Geometry: final body of the model. Coordinates: model frame, mm. Face numbers are marked on the shaded views. Coordinates: 2 decimals unless noted, no trailing zeros. Order: outer loops, then holes, each group sorted by start corner. A loop starts at its lowest first (then second) coordinate and runs counter-clockwise, first axis right, second up. Notation, with made-up numbers: M 25.25,0 L 34.25,0 A12 cw 34.25,18 Z; hole C 76.25,3 d3. An arc over 180 degrees is marked long. Write item = value, one per line.
from build123d import *

# Parameters (mm, degrees)
BOSS_EXTRUDE3_DEPTH = 7.8
SKETCH2_R           = 2.4
CUT_EXTRUDE1_DEPTH  = 7.8
SKETCH3_R           = 3.05
CUT_EXTRUDE2_DEPTH  = 0.8
SKETCH4_R           = 3.05
CUT_EXTRUDE3_DEPTH  = 0.8


with BuildPart() as part:
    # Sketch1 → Boss-Extrude3 (new body)
    with BuildSketch(Plane(origin=(0, 0, 0), x_dir=(1, 0, 0), z_dir=(0, 1, 0))):
        with BuildLine():
            Line((-16, -3.7), (32, -3.7))
            ThreePointArc((32, -3.7), (35.7, 0), (32, 3.7))
            Line((32, 3.7), (-16, 3.7))
            ThreePointArc((-16, 3.7), (-19.7, 0), (-16, -3.7))
        make_face()
    extrude(amount=BOSS_EXTRUDE3_DEPTH)

    # Sketch2 → Cut-Extrude1 (cut)
    with BuildSketch(Plane(origin=(0, 7.8, 0), x_dir=(1, 0, 0), z_dir=(0, 1, 0))):
        Circle(SKETCH2_R)
        with Locations((8, 0)):
            Circle(SKETCH2_R)
        with Locations((16, 0)):
            Circle(SKETCH2_R)
        with Locations((-16, 0)):
            Circle(SKETCH2_R)
        with Locations((-8, 0)):
            Circle(SKETCH2_R)
        with Locations((24, 0)):
            Circle(SKETCH2_R)
        with Locations((32, 0)):
            Circle(SKETCH2_R)
    extrude(amount=-CUT_EXTRUDE1_DEPTH, mode=Mode.SUBTRACT)

    # Sketch3 → Cut-Extrude2 (cut)
    with BuildSketch(Plane(origin=(0, 7.8, 0), x_dir=(1, 0, 0), z_dir=(0, 1, 0))):
        Circle(SKETCH3_R)
        with Locations((8, 0)):
            Circle(SKETCH3_R)
        with Locations((16, 0)):
            Circle(SKETCH3_R)
        with Locations((-16, 0)):
            Circle(SKETCH3_R)
        with Locations((-8, 0)):
            Circle(SKETCH3_R)
        with Locations((32, 0)):
            Circle(SKETCH3_R)
        with Locations((24, 0)):
            Circle(SKETCH3_R)
    extrude(amount=-CUT_EXTRUDE2_DEPTH, mode=Mode.SUBTRACT)

    # Sketch4 → Cut-Extrude3 (cut)
    with BuildSketch(Plane.XZ):
        Circle(SKETCH4_R)
        with Locations((8, 0)):
            Circle(SKETCH4_R)
        with Locations((16, 0)):
            Circle(SKETCH4_R)
        with Locations((-16, 0)):
            Circle(SKETCH4_R)
        with Locations((-8, 0)):
            Circle(SKETCH4_R)
        with Locations((32, 0)):
            Circle(SKETCH4_R)
        with Locations((24, 0)):
            Circle(SKETCH4_R)
    extrude(amount=-CUT_EXTRUDE3_DEPTH, mode=Mode.SUBTRACT)


solid = part.part
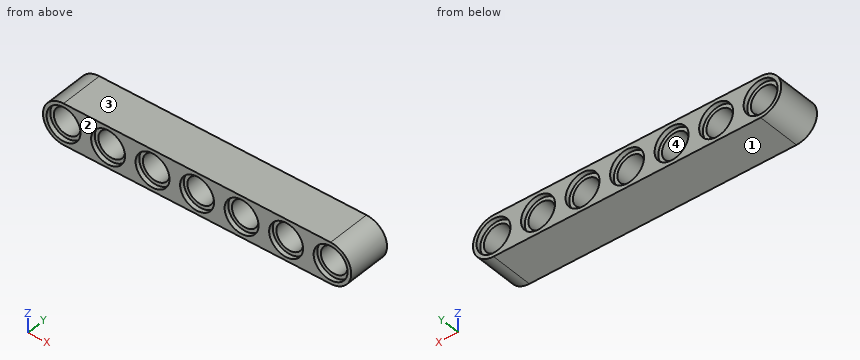
1) Mould query, pull axis Z, two halves, no side actions, for the marked faces 1, 2, 3 and 4. Classes: pulls with the +Z half, pulls with the -Z half, needs draft (parallel to the pull), parting line crosses it, or undercut.
Numbers:
face_1 = pulls with the -Z half
face_2 = needs draft
face_3 = pulls with the +Z half
face_4 = undercut
2) Section A-A, the plane y = 5.75. Return loops of the section in (x, z).
Numbers:
outline = M -16,-3.7 L 32,-3.7 A3.7 ccw 32,3.7 L -16,3.7 A3.7 ccw Z; hole C -16,0 d4.8; hole C -8,0 d4.8; hole C 0,0 d4.8; hole C 8,0 d4.8; hole C 16,0 d4.8; hole C 24,0 d4.8; hole C 32,0 d4.8
3) Section D-D, the plane x = 1. Return loops of the section in (y, z).
Numbers:
outline = M 0,-3.7 L 7.8,-3.7 L 7.8,-2.88 L 7,-2.88 L 7,-2.18 L 0.8,-2.18 L 0.8,-2.88 L 0,-2.88 Z; M 0,2.88 L 0.8,2.88 L 0.8,2.18 L 7,2.18 L 7,2.88 L 7.8,2.88 L 7.8,3.7 L 0,3.7 Z
4) Line query: L1, parallel to Z at x = 0, y = 7.45; L2, parallel to Z at x = 8, y = 1.5; L3, parallel to Y at x = -15, z = -2.5. Output: solid intervals per line, ascending.
Numbers:
L1 = -3.7 to -3.05, 3.05 to 3.7
L2 = -3.7 to -2.4, 2.4 to 3.7
L3 = 0.8 to 7
5) Pin query (flat end, axial travel): pin 1 (1 mm diameter, centred on y = 1.5, z = -1, fed in from +X); pin 2 (1.5 mm diameter, centred on y = 7, z = 1.5, fed in from +X); pin 3 (3 mm diameter, centred on y = 5, z = 2.5, fed in from -X). Return the tip coordinate at first contact, or that it passes through.
Numbers:
pin_1 = 35.67
pin_2 = 35.62
pin_3 = -19.56
6) Section B-B, the plane x = 24. Return loops of the section in (y, z), and give its area (3 significant figures).
Numbers:
outline = M 0,-3.7 L 7.8,-3.7 L 7.8,-3.05 L 7,-3.05 L 7,-2.4 L 0.8,-2.4 L 0.8,-3.05 L 0,-3.05 Z; M 0,3.05 L 0.8,3.05 L 0.8,2.4 L 7,2.4 L 7,3.05 L 7.8,3.05 L 7.8,3.7 L 0,3.7 Z
area = 18.2 mm²
7) Section C-C, the plane z = 0. Give the number of separate pieces and of enclosed holes in the cut face, and give its area (3 significant figures).
Numbers:
separate_pieces = 8
enclosed_holes = 0
area = 155 mm²
